Can you work these out from the model? Positions are in its coordinate system, mm. Face numbers are marked on the shaded views. Give positions to 0.01 mm unless a question says otherwise; leave off trailing zeros. Loops run counter-clockwise (first coordinate to the right, second up) from the corner with the lowest first, then second, coordinate; pieces in that order, holes last. Notation, with made-up numbers: (62, -33.75) - (101, -33.75) arc R21 cw to (101, -7.75) - close; hole circle Ø4 at (1.5, -17.75). An arc over 180 degrees is marked (long way). Use a Markdown table: item, result. Add a question column.
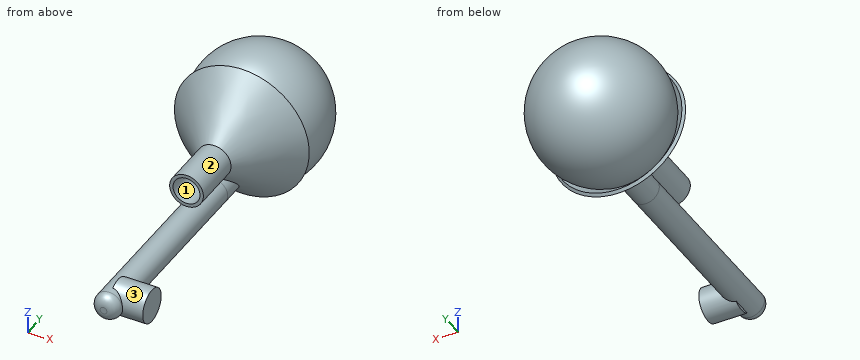
```python
from build123d import *

# Parameters (mm, degrees)
BOSS_EXTRUDE1_REACH             = 46.32
SKETCH2_R                       = 4
BOSS_EXTRUDE1_DIRECTION_2_DEPTH = 60
FILLET1_R                       = 3
SKETCH3_R                       = 5
BOSS_EXTRUDE2_DEPTH             = 10


with BuildPart() as part:
    # Sketch1 → Revolve1 (revolve)
    with BuildSketch(Plane.XY):
        with BuildLine():
            Line((-5, 0), (-5, -15))
            Line((-5, -15), (-4, -15))
            Line((-4, -15), (-4, 0))
            Line((-4, 0), (0, 0))
            Line((0, 0), (0, 44.319820094))
            ThreePointArc((0, 44.319820094), (-17.789448167, 33.459597657), (-16.259159922, 12.673373485))
            Line((-16.259159922, 12.673373485), (-19.292893219, 15.707106781))
            Line((-19.292893219, 15.707106781), (-20, 15))
            Line((-20, 15), (-5, 0))
        make_face()
    revolve(axis=Axis((0, 0, 0), (0, 1, 0)))

    # Sketch2 → Boss-Extrude1 (add, up to next)
    with BuildSketch(Plane(origin=(0, 0, 0), x_dir=(1, 0, 0), z_dir=(0, 1, 0)), mode=Mode.PRIVATE) as boss_extrude1_sk1:
        with Locations((0, 9.747716973)):
            Circle(SKETCH2_R)
    boss_extrude1_tool1 = extrude(boss_extrude1_sk1.sketch, amount=BOSS_EXTRUDE1_REACH, mode=Mode.PRIVATE) - part.part
    add(boss_extrude1_tool1.solids().sort_by_distance((0, 0, -9.747717))[0])

    # Sketch2 → Boss-Extrude1 direction 2 (add)
    with BuildSketch(Plane(origin=(0, 0, 0), x_dir=(1, 0, 0), z_dir=(0, 1, 0))):
        with Locations((0, 9.747716973)):
            Circle(SKETCH2_R)
    extrude(amount=-BOSS_EXTRUDE1_DIRECTION_2_DEPTH)

    # Fillet1
    fillet1_edges = [part.edges().sort_by_distance(p)[0] for p in [
        (-4, -60, -9.747716973),
    ]]
    fillet(fillet1_edges, radius=FILLET1_R)

    # Sketch3 → Boss-Extrude2 (add)
    with BuildSketch(Plane(origin=(0, 0, 0), x_dir=(0, 0, -1), z_dir=(1, 0, 0))):
        with Locations((9.747716973, -52)):
            Circle(SKETCH3_R)
    extrude(amount=BOSS_EXTRUDE2_DEPTH)


solid = part.part
```
1. Suppose I cut it at C-C (y = -19.5). List the corners of the cut face in (x, z) for me, and give its area (3 significant figures).
2. Suppose I cut it at A-A (y = -52). List the corners of the cut face in (x, z) for me.
3. Suppose I cut it at B-B (z = 0). List the corners of the cut face in (x, y) for me.
4. Will these pins go through, and if not, where does the flat tip stop? P1, Ø3, axis at y = -14, z = -6.5, coming from the +X side; P2, Ø1, axis at x = -3.5, z = 15, coming from the +Y side; P3, Ø3, axis at x = 5.5, z = -4.5, coming from the -Y side.
5. Please list where these lines run through material, in increasing order: line 1 along Z through (x, y) = (0, -6); line 2 along Y through (x, z) = (15, 4); line 3 along Y through (x, z) = (0.5, 10.5). Write a range as [from, to].
6. If we mould it in two halves opening along Z, with no side actions, what happens to the marked faces 1, 2 and 3? For each: released by +Z, released by -Z, zero draft, split by the parting line, or undercut.
Results below:
| question | item | result |
|---|---|---|
| 1 | outline | circle Ø8 at (0, -9.75) |
| 1 | area | 50.3 mm² |
| 2 | outline | (0, -14.75) - (10, -14.75) - (10, -4.75) - (0, -4.75) - (0, -5.75) arc R4 ccw to (0, -13.75) - close |
| 3 | outline | (-20, 15) - (-5, 0) - (-5, -15) - (-4, -15) - (-4, 0) - (4, 0) - (4, -15) - (5, -15) - (5, 0) - (20, 15) - (19.29, 15.71) - (16.26, 12.67) arc R20 ccw (long way) to (-16.26, 12.67) - (-19.29, 15.71) - close |
| 4 | P1 | x = 3.6 |
| 4 | P2 | y = 37.66 |
| 4 | P3 | y = -55.31 |
| 5 | line 1 | [-13.75, -5.75], [-5, -4], [4, 5] |
| 5 | line 2 | [10.52, 36.93] |
| 5 | line 3 | [5.51, 41.33] |
| 6 | face 1 | undercut |
| 6 | face 2 | undercut |
| 6 | face 3 | split by the parting line |
